Autodesk Fusion 360 part; units mm, degrees
sketch "Sketch1" plane through (0, 0, 0) normal (0, 0, 1) x (1, 0, 0)
  line L0 (0, 0) -> (10.16, 0)
  line L1 (10.16, 0) -> (10.16, 10.16)
  line L2 (10.16, 10.16) -> (0, 10.16)
  line L3 (0, 10.16) -> (0, 0)
  circle A0 centre (6.604, 5.08) radius 1.016
  circle A1 centre (-3.81, -4.3942) radius 1.016
  line L4 (7.6211, 0) -> (-0.6691, -8.2902)
  line L5 (7.6211, 0) -> (20.9233, 0) construction
  line L6 (-3.3632, -9.4061) -> (-5.0642, -9.4061)
  line L7 (-8.8742, -5.5961) -> (-8.8742, -1.5782)
  line L8 (-7.7583, 1.1159) -> (0, 8.8742)
  arc A2 (-3.3632, -9.4061) -> (-0.6691, -8.2902) centre (-3.3632, -5.5961) ccw
  arc A3 (-8.8742, -5.5961) -> (-5.0642, -9.4061) centre (-5.0642, -5.5961) ccw
  arc A4 (-7.7583, 1.1159) -> (-8.8742, -1.5782) centre (-5.0642, -1.5782) ccw
  dimension "d1" = 10.16
  dimension "d2" = 10.16
  dimension "d3" = 2.032
  dimension "d4" = 3.556
  dimension "d5" = 5.08
  dimension "d6" = 2.032
  dimension "d7" = 4.3942
  dimension "d8" = 3.81
  dimension "d9" = 135
  dimension "d10" = 135
  dimension "d11" = 3.81
  dimension "d12" = 3.81
  dimension "d13" = 3.81
extrude "Extrude1" add sketch "Sketch1" along normal blind 19.3294 contours L0 L1 L2 L3
extrude "Extrude2" add sketch "Sketch1" along normal blind 6.604 contours L0 L3 L4 L6 L7 L8 A2 A3 A4
extrude "Extrude3" add sketch "Sketch1" along normal blind 6.604 contours A1
extrude "Extrude4" cut sketch "Sketch1" along normal blind 5.588 contours A1
extrude "Extrude5" add sketch "Sketch1" along normal blind 12.7 contours A0
Geometry: final body of the model. Coordinates: model frame, mm. A direction names the side the tool comes from. Round coordinates to 2 decimals unless told otherwise and drop trailing zeros. Order: outer loops, then holes, each group sorted by start corner. A loop starts at its lowest first (then second) coordinate and runs counter-clockwise, first axis right, second up. Notation, with made-up numbers: M 5,12 L 16,12 A35 ccw 16,45 Z; hole C -40,52.25 d5. An arc over 180 degrees is marked long. One line per item, written item: value.
(1) Reachability of faces 4 (the flat face through (7, 5, 12.7)), 5 (the flat face through (-4, -4, 5.588)), 6 (the flat face through (5, 10.16, 10)) from +Z, -Z, +X, -X, +Y, -Y: full face, straight path, thin tool, end or side. Return the list, or none.
Result sheet:
face 4: +Z
face 5: -Z
face 6: +Z, -Z, +X, -X, +Y
(2) Cut plane B-B (x = -3.81). Return the cut outline in (y, z).
Result sheet:
outline: M -9.41,0 L -5.41,0 L -5.41,5.59 L -3.38,5.59 L -3.38,0 L 5.06,0 L 5.06,6.6 L -9.41,6.6 Z
(3) Cut plane A-A (z = 6). Return the cut outline in (x, y).
Result sheet:
outline: M -8.87,-5.6 A3.81 ccw -5.06,-9.41 L -3.36,-9.41 A3.81 ccw -0.67,-8.29 L 7.62,0 L 10.16,0 L 10.16,10.16 L 0,10.16 L 0,8.87 L -7.76,1.12 A3.81 ccw -8.87,-1.58 Z
(4) Line query: probe 1 along X at (y, z) = (-4.75, 5); probe 2 along Y at (x, z) = (-3.81, 1.9); probe 3 along Z at (x, y) = (-0.5, 0.75). Output: solid intervals per line, ascending. Write a range as [from, to].
Result sheet:
probe 1: [-8.87, -4.76], [-2.86, 2.87]
probe 2: [-9.41, -5.41], [-3.38, 5.06]
probe 3: [0, 6.6]
(5) Cut plane D-D (y = 5.08). Return the cut outline in (x, z).
Result sheet:
outline: M -3.79,0 L 10.16,0 L 10.16,19.33 L 7.62,19.33 L 7.62,12.7 L 5.59,12.7 L 5.59,19.33 L 0,19.33 L 0,6.6 L -3.79,6.6 Z
(6) Pin query (flat end, axial travel): P1, Ø8, axis at y = 7.5, z = 5, coming from the -X side; P2, Ø1, axis at x = 6, y = -2.5, coming from the -Z side; P3, Ø1.6, axis at x = -3.81, y = -4.39, coming from the -Z side; P4, Ø10, axis at x = 5.5, y = -5.5, coming from the +Z side. Return the tip coordinate at first contact, or that it passes through.
Result sheet:
P1: x = -5.37
P2: through
P3: z = 5.59
P4: z = 6.6
(7) Cut plane C-C (z = 17.25). Return the cut outline in (x, y).
Result sheet:
outline: M 0,0 L 10.16,0 L 10.16,10.16 L 0,10.16 Z; hole C 6.6,5.08 d2.03
(8) Pull-direction query (X, two-part tool) for faces 1 (the flat face through (-8.874, -4, 3)), 2 (the flat face through (5, 5, 19.329)), 3 (the cylindrical face through (-4.62, -3.78, 2.75)); classes: pulls with the +X half, pulls with the -X half, needs draft (parallel to the pull), parting line crosses it, or undercut.
Result sheet:
face 1: pulls with the -X half
face 2: needs draft
face 3: undercut
